For this review, take the finished solid that the model builds, in its own axes (mm). Round coordinates to 2 decimals unless told otherwise and drop trailing zeros. Order: outer loops, then holes, each group sorted by start corner. A loop starts at its lowest first (then second) coordinate and runs counter-clockwise, first axis right, second up. Notation, with made-up numbers: M 69,7.25 L 93,7.25 A10 ccw 93,25.25 Z; hole C -38.75,-35 d11. An arc over 180 degrees is marked long. Use a Markdown table: item, result.
Autodesk Inventor part; units mm, degrees
ref_plane "YZ Plane" through (0, 0, 0) normal (1, 0, 0) x (0, 1, 0)
ref_plane "XZ Plane" through (0, 0, 0) normal (0, 1, 0) x (-1, 0, 0)
ref_plane "XY Plane" through (0, 0, 0) normal (0, 0, 1) x (1, 0, 0)
sketch "Sketch1" plane through (0, 0, 0) normal (0, 1, 0) x (-1, 0, 0)
  line L0 (25, 100) -> (-25, 100)
  line L1 (-25, 100) -> (-25, -100)
  line L2 (-25, -100) -> (25, -100)
  line L3 (25, -100) -> (25, 100)
  line L4 (25, 100) -> (-25, -100) construction
  line L5 (-25, 100) -> (25, -100) construction
  point P0 (0, 0)
  dimension "d0" = 50
  dimension "d1" = 200
extrude "Extrusion1" add sketch "Sketch1" along normal blind 62
sketch "Sketch2" plane through (-25, 0, 100) normal (0, 0, 1) x (1, 0, 0)
  line L0 (50, 62) -> (0, 62)
  line L1 (50, 62) -> (90, 62)
  line L2 (90, 62) -> (90, 42)
  line L3 (90, 42) -> (53.2289, 0)
  line L4 (53.2289, 0) -> (50, 0)
  line L5 (50, 62) -> (50, 0)
  point P0 (25, 0)
  dimension "d4" = 40
  dimension "d5" = 20
  dimension "d6" = 90
extrude "Extrusion2" add sketch "Sketch2" against normal up to surface (200 mm away)
sketch "Sketch3" plane through (0, 62, 0) normal (0, 1, 0) x (1, 0, 0)
  line L0 (-25, 100) -> (-25, -100)
  line L1 (-25, -100) -> (-25, 100)
  line L2 (-25, 100) -> (-25, 80)
  line L3 (-25, 80) -> (-76.9615, 50)
  line L4 (-25, -100) -> (-25, -80)
  line L5 (-25, -80) -> (-76.9615, -50)
  line L6 (-76.9615, -50) -> (-76.9615, 50)
  circle A0 centre (-76.9615, 0) radius 49.9974
  circle A1 centre (-126.9564, -0.5064) radius 49.9974
  line L7 (-76.9615, -50) -> (-126.45, -50.5013)
  line L8 (-127.4628, 49.4885) -> (-76.9615, 50)
  point P0 (0, 0)
  point P1 (-76.9615, 49.9974)
  point P2 (-77.4679, 49.9949)
  point P3 (-76.9615, -1.0128)
  dimension "d9" = 20
  dimension "d10" = 60
  dimension "d11" = 120
  dimension "d12" = 20
  dimension "d13" = 60
  dimension "d14" = 120
extrude "Extrusion3" add sketch "Sketch3" against normal blind 62
sketch "Sketch4" plane through (0, 62, 0) normal (0, 1, 0) x (1, 0, 0)
  line L0 (-25, -100) -> (28.2289, -100)
  line L1 (-25, 100) -> (-25, 80)
  line L2 (-25, -100) -> (-25, 100)
  line L3 (-25, 100) -> (29.4775, 197.567)
  line L4 (29.4775, 197.567) -> (135.6867, 127.811)
  line L5 (135.6867, 127.811) -> (135.6867, -104.409)
  line L6 (135.6867, -104.409) -> (110.0345, -245.7212)
  line L7 (110.0345, -245.7212) -> (-5.1754, -156.6135)
  line L8 (-5.1754, -156.6135) -> (-25, -100)
  line L9 (-76.9615, -50) -> (-76.9615, 49.9974)
  line L10 (-76.9615, 49.9974) -> (-143.8651, 145.0549)
  line L11 (-143.8651, 145.0549) -> (-248.9816, -0.0013)
  line L12 (-248.9816, -0.0013) -> (-240.1494, -166.1828)
  line L13 (-240.1494, -166.1828) -> (-110.4133, -169.4443)
  line L14 (-110.4133, -169.4443) -> (-76.9615, -50)
  line L15 (-110.4133, -169.4443) -> (-5.1754, -156.6135)
  line L16 (-143.8651, 145.0549) -> (29.4775, 197.567)
  point P0 (0, 0)
extrude "Extrusion4" cut sketch "Sketch4" against normal blind 62 contours L10 L9 L14 L13 L12 L11
extrude "Extrusion5" cut sketch "Sketch4" against normal blind 62 contours L1 L2 L8 L15 L14 L9 L10 L16 L3
properties part number "piece1" material "Acrylic, Clear"
Q1. Wall thickness on line 1 along Y through (x, z) = (56, 15); line 2 along X through (y, z) = (28, 57); line 3 along X through (y, z) = (38.5, 72): over which ranges is each line inside the solid? List them lowest first. Write a range as [from, to].
Determined:
| item | result |
|---|---|
| line 1 | y = [31.72, 62] |
| line 2 | x = [-25, 52.74] |
| line 3 | x = [-25, 61.94] |
Q2. Add section C-C (x = 55.5). Write out the cut boundary in (y, z).
Determined:
| item | result |
|---|---|
| outline | M 31.15,-100 L 62,-100 L 62,100 L 31.15,100 Z |
Q3. Clearance check with a flat-ended pin moving along its axis: pin 1 (6 mm diameter, centred on x = -9.5, z = 55, fed in from -Y). State where the tip first meets the part, or that it passes through.
Determined:
| item | result |
|---|---|
| pin 1 | stops at y = 0 |
Q4. Add section B-B (y = 35.5). Write out the cut boundary in (x, z), then the cut area to 3 significant figures.
Determined:
| item | result |
|---|---|
| outline | M -25,-100 L 59.31,-100 L 59.31,100 L -25,100 Z |
| area | 16,900 mm^2 |
Q5. Add section A-A (z = 10). Write out the cut boundary in (x, y).
Determined:
| item | result |
|---|---|
| outline | M -25,0 L 28.23,0 L 65,42 L 65,62 L -25,62 Z |
